Source: CAD feature listing. Evaluate the final solid. Frame: model axes, mm. A direction names the side the tool comes from. Round coordinates to 2 decimals unless told otherwise and drop trailing zeros. Loops run counter-clockwise (first coordinate to the right, second up) from the corner with the lowest first, then second, coordinate; pieces in that order, holes last. Notation, with made-up numbers: M 39,72 L 74,72 A10 cw 74,90 Z; hole C 45.5,89.5 d6. An arc over 180 degrees is marked long. Answer as a JSON object with one key per item and string values.
from build123d import *

# Parameters (mm, degrees)
SKETCH1_W           = 133.5
SKETCH1_H           = 46
SKETCH1_R           = 10
SKETCH1_R_2         = 7
BOSS_EXTRUDE1_DEPTH = 12
SKETCH2_R           = 11
CUT_EXTRUDE1_DEPTH  = 5
M4_TAPPED_HOLE1_D   = 3.3


with BuildPart() as part:
    # Sketch1 → Boss-Extrude1 (new body)
    with BuildSketch(Plane.XY):
        Rectangle(SKETCH1_W, SKETCH1_H)
        with Locations((50, 0)):
            Circle(SKETCH1_R, mode=Mode.SUBTRACT)
        with Locations((-50, 0)):
            Circle(SKETCH1_R, mode=Mode.SUBTRACT)
        Circle(SKETCH1_R_2, mode=Mode.SUBTRACT)
    extrude(amount=BOSS_EXTRUDE1_DEPTH)

    # Sketch2 → Cut-Extrude1 (cut)
    with BuildSketch(Plane(origin=(0, 0, 0), x_dir=(-1, 0, 0), z_dir=(0, 0, -1))):
        Circle(SKETCH2_R)
    extrude(amount=-CUT_EXTRUDE1_DEPTH, mode=Mode.SUBTRACT)

    # M4 Tapped Hole1 (through all)
    with Locations(Plane.ZY.offset(66.75)):
        with Locations((6, 12), (6, -12)):
            m4_tapped_hole1 = Hole(M4_TAPPED_HOLE1_D / 2)

    # Mirror1: M4 Tapped Hole1 across plane
    add(m4_tapped_hole1.mirror(Plane(origin=(0, 0, 0), x_dir=(0, 0, 1), z_dir=(1, 0, 0))), mode=Mode.SUBTRACT)


solid = part.part
Item 1: Section C-C on x = -13. Return the cut outline in (y, z), then the cut area to 3 significant figures.
Answer sheet:
{"outline": "M -23,0 L 23,0 L 23,12 L -23,12 Z; hole C -12,6 d3.3; hole C 12,6 d3.3", "area": "535 mm²"}
Item 2: Section D-D on x = 1. Return the cut outline in (y, z).
Answer sheet:
{"outline": "M -23,0 L -10.95,0 L -10.95,4.72 A1.65 cw long -10.69,5 L -6.93,5 L -6.93,12 L -23,12 Z; M 6.93,5 L 10.69,5 A1.65 cw long 10.95,4.72 L 10.95,0 L 23,0 L 23,12 L 6.93,12 Z"}
Item 3: Pull-direction query (Y, two-part tool) for faces 3 (the flat face through (66.75, 0, 6)), 4 (the cylindrical face through (0.93, -13, 7.31)), 5 (the flat face through (-1, -23, 6)), 6 (the flat face through (-1, 23, 6)); classes: pulls with the +Y half, pulls with the -Y half, needs draft (parallel to the pull), parting line crosses it, or undercut.
Answer sheet:
{"face 3": "needs draft", "face 4": "undercut", "face 5": "pulls with the -Y half", "face 6": "pulls with the +Y half"}
Item 4: Line query: probe 1 along X at (y, z) = (-0.5, 4.25); probe 2 along Y at (x, z) = (32, 6.75); probe 3 along Y at (x, z) = (-50, 4.5). Output: solid intervals per line, ascending. Write a range as from..to.
Answer sheet:
{"probe 1": "x = -66.75..-59.99, -40.01..-10.99, 10.99..40.01, 59.99..66.75", "probe 2": "y = -23..-13.47, -10.53..10.53, 13.47..23", "probe 3": "y = -23..-12.69, -11.31..-10, 10..11.31, 12.69..23"}
Item 5: Section A-A on x = -50. Return the cut outline in (y, z).
Answer sheet:
{"outline": "M -23,0 L -10,0 L -10,12 L -23,12 Z; M 10,0 L 23,0 L 23,12 L 10,12 Z; hole C -12,6 d3.3; hole C 12,6 d3.3"}
Item 6: Section B-B on y = 3. Return the cut outline in (x, z).
Answer sheet:
{"outline": "M -66.75,0 L -59.54,0 L -59.54,12 L -66.75,12 Z; M -40.46,0 L -10.58,0 L -10.58,5 L -6.32,5 L -6.32,12 L -40.46,12 Z; M 6.32,5 L 10.58,5 L 10.58,0 L 40.46,0 L 40.46,12 L 6.32,12 Z; M 59.54,0 L 66.75,0 L 66.75,12 L 59.54,12 Z"}
Item 7: Contact query for flat-ended pins moving along their axis: pin 1 Ø3 at (y, z) = (12, 6) entering from +X; pin 2 Ø17 at (x, y) = (-4, -3) entering from -Z. Output: stop coordinate, or through.
Answer sheet:
{"pin 1": "passes through", "pin 2": "stops at z = 0"}
Item 8: Access query for faces 1 (the cylindrical face through (2.38, -10.74, 2.46)), 2 (the flat face through (-1, 11, 12)). Directions: +Z, -Z, +X, -X, +Y, -Y. A direction counts if a zero-diameter tool reaches every point of the face in a straight line with its end or side. Return the directions, or none.
Answer sheet:
{"face 1": "-Z", "face 2": "+Z, +X, -X, +Y, -Y"}
